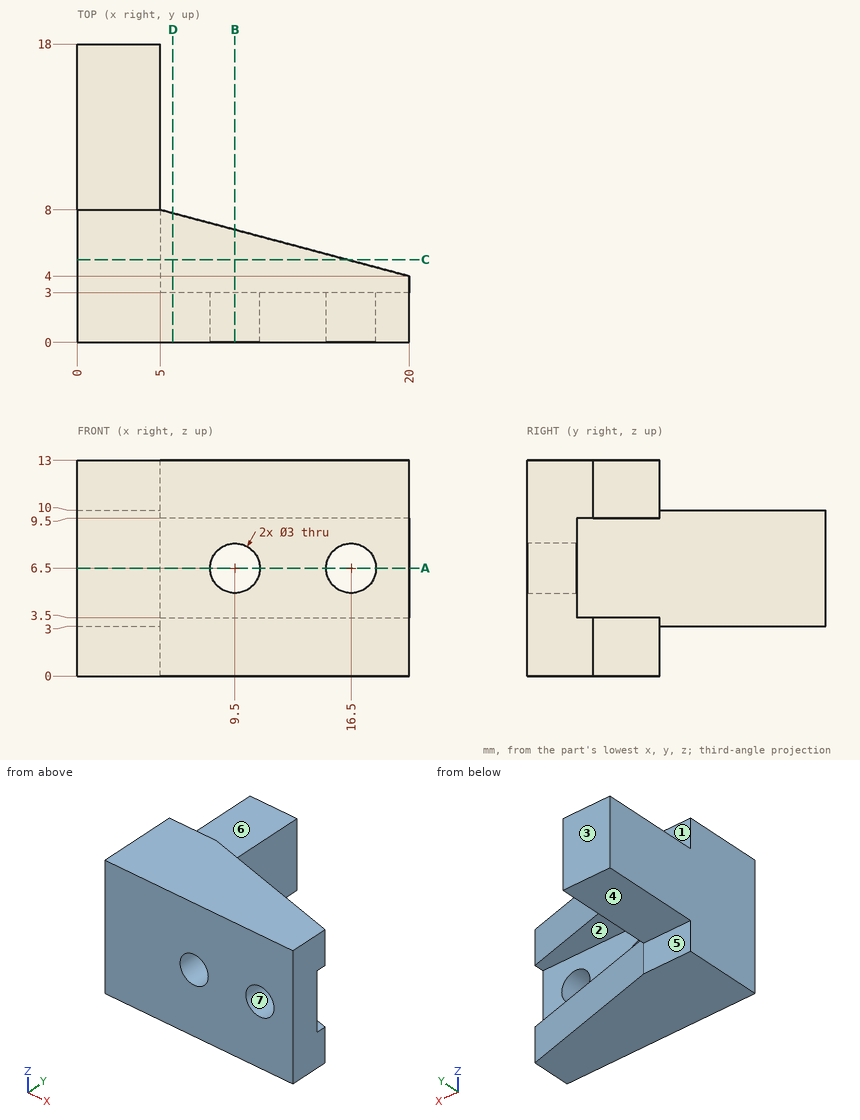
Answer from the drawing. Dimensions are ordinates in mm from the lowest x, y and z of the part. A direction names the side the tool comes from. Coordinates: 2 decimals unless noted, no trailing zeros. Order: outer loops, then holes, each group sorted by start corner. A loop starts at its lowest first (then second) coordinate and runs counter-clockwise, first axis right, second up. Notation, with made-up numbers: (5, 68.25) - (41, 68.25) arc R22 cw to (41, 83.25) - close; hole circle Ø6 at (23, 75.25). An arc over 180 degrees is marked (long way). Put each result on its own line as item: value. Start each with the question number.
1) For the marked faces 1, 2 and 3, determine the directions among +Z, -Z, +X, -X, +Y, -Y from which every point of the face is accessible in a straight line to the end or side of a thin tool.
2) Find section A-A (z = 6.5). Give the vertices of the cut face in (x, y), plus the area to 3 significant figures.
3) Flat-ended cylindrical pins translate along their axes: pin 1 (3.5 mm diameter, centred on x = 16.5, z = 6.5, fed in from +Y); pin 2 (3.5 mm diameter, centred on x = 2, z = 12, fed in from +Y); pin 3 (5.5 mm diameter, centred on x = 3, y = 14, fed in from +Z). Find the tip coordinate at first contact, or state that the pin passes through.
4) Find section C-C (y = 5). Give the vertices of the cut face in (x, z).
5) For a pull along Z with two mould halves and no side action, classify the marked faces 4, 5, 6 and 7 as released by +Z, released by -Z, zero draft, split by the parting line, or undercut.
6) Find section B-B (x = 9.5). Give the vertices of the cut face in (y, z), plus the area to 3 significant figures.
7) Find section D-D (x = 5.75). Give the vertices of the cut face in (y, z), plus the area to 3 significant figures.
8) Find the intervals of material crossed by line 1 (X direction, y = 0.9, z = 6.5); line 2 (Z direction, x = 16, y = 5); line 3 (X direction, y = 3.5, z = 7.25), in increasing order. Write a range as from..to.
Results list:
1. face 1: +Z, +X, -X, +Y
1. face 2: +X, +Y
1. face 3: +Z, -Z, +X, -X, +Y
2. outline: (0, 0) - (8, 0) - (8, 3) - (5, 3) - (5, 18) - (0, 18) - close; (11, 0) - (15, 0) - (15, 3) - (11, 3) - close; (18, 0) - (20, 0) - (20, 3) - (18, 3) - close
2. area: 117 mm^2
3. pin 1: stops at y = 3
3. pin 2: stops at y = 8
3. pin 3: stops at z = 10
4. outline: (0, 0) - (16.25, 0) - (16.25, 3.5) - (5, 3.5) - (5, 9.5) - (16.25, 9.5) - (16.25, 13) - (0, 13) - close
5. face 4: released by -Z
5. face 5: zero draft
5. face 6: released by +Z
5. face 7: undercut
6. outline: (0, 0) - (6.8, 0) - (6.8, 3.5) - (3, 3.5) - (3, 5) - (0, 5) - close; (0, 8) - (3, 8) - (3, 9.5) - (6.8, 9.5) - (6.8, 13) - (0, 13) - close
6. area: 56.6 mm^2
7. outline: (0, 0) - (7.8, 0) - (7.8, 3.5) - (3, 3.5) - (3, 9.5) - (7.8, 9.5) - (7.8, 13) - (0, 13) - close
7. area: 72.6 mm^2
8. line 1: x = 0..8, 11..15, 18..20
8. line 2: z = 0..3.5, 9.5..13
8. line 3: x = 0..5
